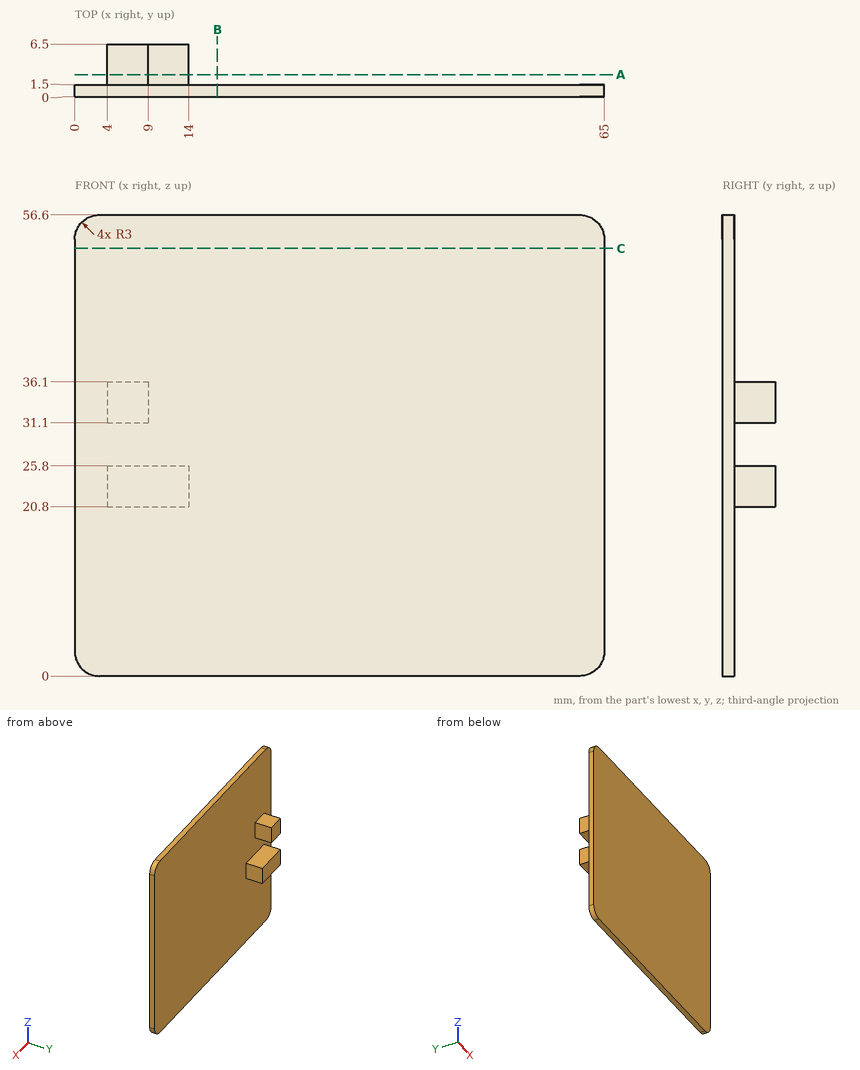
Answer from the drawing. Dimensions are ordinates in mm from the lowest x, y and z of the part. Give positions to 0.01 mm unless a question says otherwise; leave off trailing zeros. Order: outer loops, then holes, each group sorted by start corner. A loop starts at its lowest first (then second) coordinate and runs counter-clockwise, first axis right, second up.
Item 1: The part is cut by section B-B, the plane x = 17.5. Give the vertices of the cut face in (y, z), and give its area (3 significant figures).
From the geometry:
outline: (0, 0) - (1.5, 0) - (1.5, 56.6) - (0, 56.6) - close
area: 84.9 mm2
Item 2: Given pin 1 Ø6 at (x, z) = (57.5, 49) entering from +Y; pin 2 Ø1.5 at (x, y) = (11.5, 5) entering from +Z; pin 3 Ø2.5 at (x, y) = (7.5, 4) entering from +Z, each flat-ended and moving along its own axis, determine where each tip first touches the part or whether it passes through.
From the geometry:
pin 1: stops at y = 1.5
pin 2: stops at z = 25.8
pin 3: stops at z = 36.1
Item 3: The part is cut by section A-A, the plane y = 2.75. Give the vertices of the cut face in (x, z).
From the geometry:
outline: (4, 20.8) - (14, 20.8) - (14, 25.8) - (4, 25.8) - close; (4, 31.1) - (9, 31.1) - (9, 36.1) - (4, 36.1) - close
Item 4: The part is cut by section C-C, the plane z = 52.5. Give the vertices of the cut face in (x, y), and give its area (3 significant figures).
From the geometry:
outline: (0, 0) - (65, 0) - (65, 1.5) - (0, 1.5) - close
area: 97.5 mm2
Item 5: Find the intervals of material crossed by probe 1 along Z at (x, y) = (4.5, 6); probe 2 along Y at (x, z) = (56.5, 45); probe 3 along X at (y, z) = (4.25, 35), in increasing order.
From the geometry:
probe 1: z = 20.8 to 25.8, 31.1 to 36.1
probe 2: y = 0 to 1.5
probe 3: x = 4 to 9
